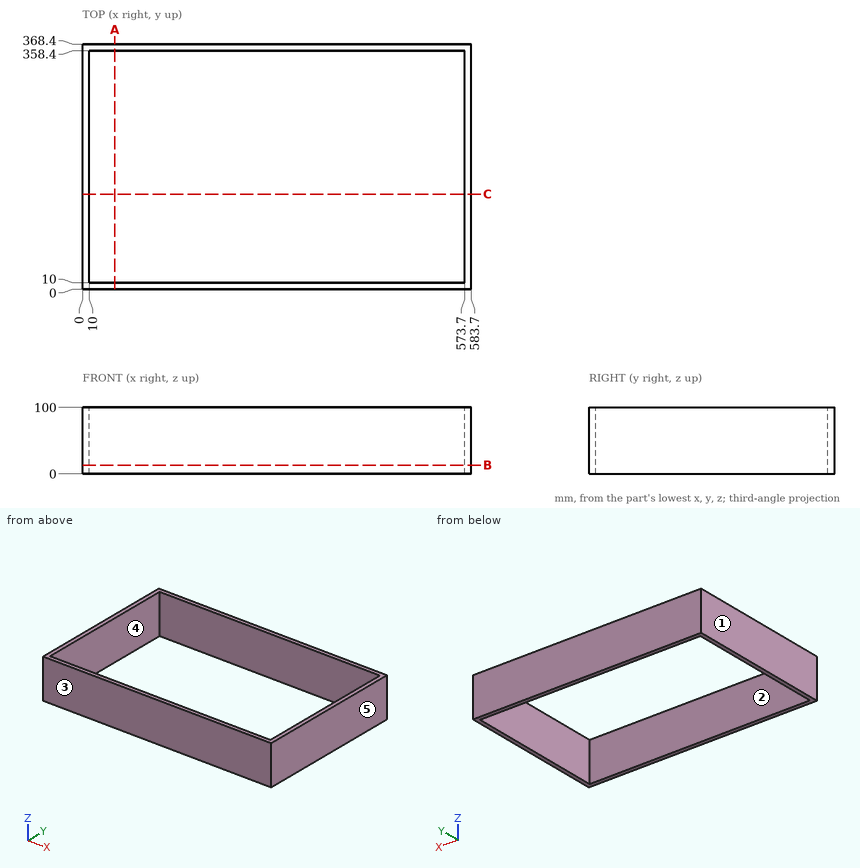
Check sheet for the drawn part. Datum: minimum x, y, z corner. Units: mm. A direction names the side the tool comes from. Round coordinates to 2 decimals unless told otherwise and drop trailing zeros. Order: outer loops, then holes, each group sorted by start corner. A loop starts at its lowest first (then second) coordinate and runs counter-clockwise, first axis right, second up.
(1) Scan lines: probe 1 along X at (y, z) = (197, 23); probe 2 along Y at (x, z) = (191.5, 26). Record each from-to range of solid material in increasing order.
(2) Cross-section at B-B, the plane z = 13. Enter the section's corners in (x, y).
(3) Cross-section at C-C, the plane y = 143. Enter the section's corners in (x, z), and give its area (3 significant figures).
(4) Cross-section at A-A, the plane x = 48.5. Enter the section's corners in (y, z).
(5) Access from +Z, -Z, +X, -X, +Y, -Y to the whole of each face (thin tool, end or side, straight path). Record for the marked faces 1 and 2.
(6) Draft check along X on the marked faces 3, 4 and 5. Enter one of: pulls with the +X half, pulls with the -X half, needs draft (parallel to the pull), parting line crosses it, or undercut.
Check sheet entries:
1. probe 1: x = 0 to 10, 573.7 to 583.7
1. probe 2: y = 0 to 10, 358.4 to 368.4
2. outline: (0, 0) - (583.7, 0) - (583.7, 368.4) - (0, 368.4) - close; hole (10, 10) - (573.7, 10) - (573.7, 358.4) - (10, 358.4) - close
3. outline: (0, 0) - (10, 0) - (10, 100) - (0, 100) - close; (573.7, 0) - (583.7, 0) - (583.7, 100) - (573.7, 100) - close
3. area: 2,000 mm2
4. outline: (0, 0) - (10, 0) - (10, 100) - (0, 100) - close; (358.4, 0) - (368.4, 0) - (368.4, 100) - (358.4, 100) - close
5. face 1: +Z, -Z, -X, +Y, -Y
5. face 2: +Z, -Z
6. face 3: needs draft
6. face 4: undercut
6. face 5: pulls with the +X half
